Build history of the part. All positions in model axes, mm. Face numbers are marked on the shaded views. A direction names the side the tool comes from. Round coordinates to 2 decimals unless told otherwise and drop trailing zeros. Loops run counter-clockwise (first coordinate to the right, second up) from the corner with the lowest first, then second, coordinate; pieces in that order, holes last. Notation, with made-up numbers: (84.5, -8.75) - (135.5, -8.75) arc R19 ccw to (135.5, 25.25) - close; hole circle Ø6 at (63, 54). An arc over 180 degrees is marked (long way). Use one line per item in the form item = value. Start each with the question number.
Q1. Drill centre lines: line 1 (Y direction, x = 17.5, z = -0.75); line 2 (Z direction, x = 12.5, y = 28.5); line 3 (X direction, y = 21, z = 1.5). Where is each one in solid material? Low to high.
Q2. Saw through at C-C (x = 13). Give the cut face in (y, z), then the cut area to 3 significant figures.
Q3. Saw through at D-D (y = -11.5). Give the cut face in (x, z).
Q4. Saw through at B-B (x = 6.5). Give the cut face in (y, z), then the cut area to 3 significant figures.
Q5. Saw through at A-A (z = -12). Give the cut face in (x, y), then the cut area to 3 significant figures.
Q6. Pin check, flat tips, straight feed: pin 1 (9 mm diameter, centred on x = 16.76, y = 5.28, fed in from +Z); pin 2 (1.5 mm diameter, centred on y = 9.5, z = 2, fed in from -X); pin 3 (12 mm diameter, centred on x = 15.5, z = -20.5, fed in from +Y); pin 4 (2.5 mm diameter, centred on y = 6.5, z = 1.5, fed in from +X). Stop position of each tip, or through.
Q7. 3-axis set-ups, long thin cutter, end or side, ignore diameter. For the marked faces 1 and 2: which of +Z, -Z, +X, -X, +Y, -Y reach the whole face in a straight line?
```python
from build123d import *

# Parameters (mm, degrees)
SALIENTE_EXTRUIR1_DEPTH = 52.5
CORTAR_EXTRUIR3_REACH   = 40.766
CROQUIS3_R              = 1.75
CROQUIS4_R              = 2.75
CORTAR_EXTRUIR4_DEPTH   = 1.5
CROQUIS5_R              = 7
SALIENTE_EXTRUIR2_DEPTH = 2.9
REDONDEO1_R             = 2


with BuildPart() as part:
    # Croquis2 → Saliente-Extruir1 (new body)
    with BuildSketch(Plane(origin=(0, 33.282514016, 0), x_dir=(1, 0, 0), z_dir=(0, 1, 0))):
        Polygon((19.664416593, -1), (19.664416593, -0.1), (2.864416593, -0.1), (2.864416593, -1), (2.864416593, -3), (19.664416593, -3), align=None)
    extrude(amount=-SALIENTE_EXTRUIR1_DEPTH)

    # Croquis3 → Cortar-Extruir3 (cut, up to next)
    with BuildSketch(Plane.XY.offset(3), mode=Mode.PRIVATE) as cortar_extruir3_sk1:
        with Locations((5.764416593, 30.282514016)):
            Circle(CROQUIS3_R)
    cortar_extruir3_tool1 = extrude(cortar_extruir3_sk1.sketch, amount=-CORTAR_EXTRUIR3_REACH, mode=Mode.PRIVATE) & part.part
    # Croquis3 → Cortar-Extruir3 (cut, up to next)
    with BuildSketch(Plane.XY.offset(3), mode=Mode.PRIVATE) as cortar_extruir3_sk2:
        with Locations((16.764416593, 5.282514016)):
            Circle(CROQUIS3_R)
    cortar_extruir3_tool2 = extrude(cortar_extruir3_sk2.sketch, amount=-CORTAR_EXTRUIR3_REACH, mode=Mode.PRIVATE) & part.part
    add(cortar_extruir3_tool1.solids().sort_by_distance((5.764417, 30.282514, 3))[0], mode=Mode.SUBTRACT)
    add(cortar_extruir3_tool2.solids().sort_by_distance((16.764417, 5.282514, 3))[0], mode=Mode.SUBTRACT)

    # Croquis4 → Cortar-Extruir4 (cut)
    with BuildSketch(Plane.XY.offset(3)):
        with Locations((5.764416593, 30.282514016)):
            Circle(CROQUIS4_R)
        with Locations((16.764416593, 5.282514016)):
            Circle(CROQUIS4_R)
    extrude(amount=-CORTAR_EXTRUIR4_DEPTH, mode=Mode.SUBTRACT)

    # Croquis5 → Saliente-Extruir2 (add)
    with BuildSketch(Plane(origin=(0, -19.217485984, 0), x_dir=(1, 0, 0), z_dir=(0, 1, 0))):
        with BuildLine():
            Line((2.864416593, -3), (19.664416593, -3))
            Line((19.664416593, -3), (22.46664072, 9.343319648))
            ThreePointArc((22.46664072, 9.343319648), (10.29394354, 23.990773749), (-0.693676229, 8.434595553))
            Line((-0.693676229, 8.434595553), (2.864416593, -3))
        make_face()
        with Locations(Location((10.764416593, 12, 0), (0, 0, 270))):
            Circle(CROQUIS5_R, mode=Mode.SUBTRACT)
    extrude(amount=SALIENTE_EXTRUIR2_DEPTH)

    # Redondeo1
    # the kernel refuses this fillet: 2 mm, written as the material it takes off along each edge
    with BuildSketch(Plane(origin=(-2.135583407, -19.217485984, 3), x_dir=(0, 1, 0), z_dir=(1, 0, 0))) as redondeo1_piece_1:
        with BuildLine():
            CenterArc((REDONDEO1_R, -REDONDEO1_R), REDONDEO1_R, 90, 90)
            Line((0, -REDONDEO1_R), (0, 0))
            Line((0, 0), (REDONDEO1_R, 0))
        make_face()
    extrude(amount=26.8, mode=Mode.SUBTRACT)
    with BuildSketch(Plane(origin=(-2.135583407, 33.282514016, 3), x_dir=(0, -1, 0), z_dir=(1, 0, 0))) as redondeo1_piece_2:
        with BuildLine():
            CenterArc((REDONDEO1_R, REDONDEO1_R), REDONDEO1_R, 180, 90)
            Line((0, REDONDEO1_R), (0, 0))
            Line((0, 0), (REDONDEO1_R, 0))
        make_face()
    extrude(amount=26.8, mode=Mode.SUBTRACT)


solid = part.part
```
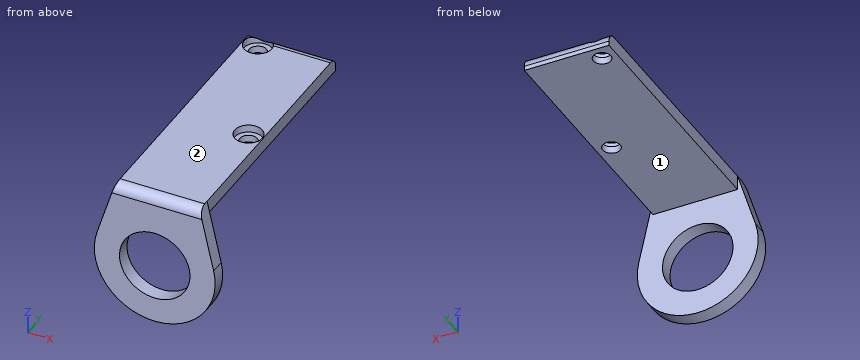
Report:
q1.line_1 = -19.22 to -16.32
q1.line_2 = 0.1 to 3
q1.line_3 = 2.86 to 19.66
q2.outline = (-19.22, -23.79) - (-16.32, -23.79) - (-16.32, -18.63) - (-19.22, -18.63) - close; (-19.22, -5.37) - (-16.32, -5.37) - (-16.32, 0.1) - (33.28, 0.1) - (33.28, 1) arc R2 ccw to (31.28, 3) - (-17.22, 3) arc R2 ccw to (-19.22, 1) - close
q2.area = 181 mm²
q3.outline = (2.86, 0.1) - (19.66, 0.1) - (19.66, 3) - (2.86, 3) - close
q4.outline = (-19.22, -23.22) - (-16.32, -23.22) - (-16.32, -17.55) - (-19.22, -17.55) - close; (-19.22, -6.45) - (-16.32, -6.45) - (-16.32, 0.1) - (28.69, 0.1) - (28.69, 1.5) - (27.63, 1.5) - (27.63, 3) - (-17.22, 3) arc R2 ccw to (-19.22, 1) - close; (31.87, 0.1) - (33.28, 0.1) - (33.28, 1) arc R2 ccw to (32.93, 2.13) - (32.93, 1.5) - (31.87, 1.5) - close
q4.area = 174 mm²
q5.outline = (-1.24, -19.22) - (3.76, -19.22) - (3.76, -16.32) - (-1.24, -16.32) - close; (17.76, -19.22) - (22.76, -19.22) - (22.76, -16.32) - (17.76, -16.32) - close
q5.area = 29.0 mm²
q6.pin_1 = 3
q6.pin_2 = 2.86
q6.pin_3 = -16.32
q6.pin_4 = 19.66
q7.face_1 = -Z, +X, -X, +Y
q7.face_2 = +Z, +X, -X, +Y, -Y
